from build123d import *

# Parameters (mm, degrees)
SALIENTE_EXTRUIR1_DEPTH = 40
CROQUIS2_R              = 3
CORTAR_EXTRUIR1_DEPTH   = 10


with BuildPart() as part:
    # Croquis1 → Saliente-Extruir1 (new body)
    with BuildSketch(Plane(origin=(0, 0, 0), x_dir=(1, 0, 0), z_dir=(0, 1, 0))):
        with BuildLine():
            Line((6.013434035, -15.633333333), (31.013434035, -15.633333333))
            Line((31.013434035, -15.633333333), (31.013434035, -12.633333333))
            Line((31.013434035, -12.633333333), (15.504802123, -12.633333333))
            ThreePointArc((15.504802123, -12.633333333), (0, 20), (-15.504802123, -12.633333333))
            Line((-15.504802123, -12.633333333), (-31.013434035, -12.633333333))
            Line((-31.013434035, -12.633333333), (-31.013434035, -15.633333333))
            Line((-31.013434035, -15.633333333), (-6.013434035, -15.633333333))
            ThreePointArc((-6.013434035, -15.633333333), (0, 16.75), (6.013434035, -15.633333333))
        make_face()
    extrude(amount=SALIENTE_EXTRUIR1_DEPTH)

    # Croquis2 → Cortar-Extruir1 (cut)
    with BuildSketch(Plane(origin=(0, 0, 12.633333333), x_dir=(-1, 0, 0), z_dir=(0, 0, -1))):
        with Locations((25.013434035, 8.154431535)):
            Circle(CROQUIS2_R)
        with Locations((25.013434035, 20.154431535)):
            Circle(CROQUIS2_R)
        with Locations((25.013434035, 32.154431535)):
            Circle(CROQUIS2_R)
        with Locations((-25.013434035, 32.154431535)):
            Circle(CROQUIS2_R)
        with Locations((-25.013434035, 8.154431535)):
            Circle(CROQUIS2_R)
        with Locations((-25.013434035, 20.154431535)):
            Circle(CROQUIS2_R)
    extrude(amount=-CORTAR_EXTRUIR1_DEPTH, mode=Mode.SUBTRACT)


solid = part.part
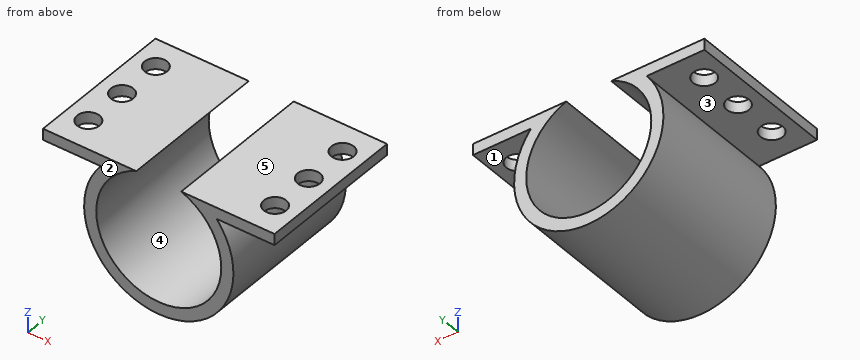
Could you check a few things on this model? Use its own coordinates, in mm. Face numbers are marked on the shaded views. A direction names the side the tool comes from. Coordinates: 2 decimals unless noted, no trailing zeros. Loops run counter-clockwise (first coordinate to the right, second up) from the corner with the lowest first, then second, coordinate; pieces in that order, holes last.
1. I need wall thicknesses on L1, parallel to X at y = 28, z = 0.5; L2, parallel to Z at x = -24.5, y = 4; L3, parallel to Z at x = 14.5, y = 15.5. Which ranges of each line are inside material? Lowest first, please.
2. For P1, Ø1.5, axis at y = 21, z = -8, coming from the +X side; P2, Ø17, axis at x = -21, y = 25.5, coming from the -Z side; P3, Ø7, axis at x = 25.01, y = 20.15, coming from the +Z side; P4, Ø5, axis at y = 25.5, z = -9, coming from the -X side, each with a flat end and sliding along its axis, tell me the tip position at first contact or that it passes through.
3. Imagine slicing it at D-D (y = 27). Please give me the cut outline in (x, z), and give its area (3 significant figures).
4. We'd pull the mould along X, two halves only. Please class the marked faces 4 and 5: released by +X, released by -X, zero draft, split by the parting line, or undercut.
5. Imagine slicing it at C-C (y = 9). Please give me the cut outline in (x, z).
6. For the marked faces 1, 2 and 3, which set-ups out of +Z, -Z, +X, -X, +Y, -Y let a thin tool reach every point of the face, with its end or its side?
7. Imagine slicing it at B-B (x = -14). Please give me the cut outline in (y, z), and give its area (3 significant figures).
8. Imagine slicing it at A-A (z = 0). Please give me the cut outline in (x, y).
Computed values:
1. L1: x = -19.99 to -16.74, 16.74 to 19.99
1. L2: z = 12.63 to 15.63
1. L3: z = -13.77 to -8.39, 8.39 to 15.63
2. P1: stops at x = 18.64
2. P2: stops at z = -15.61
2. P3: stops at z = 15.63
2. P4: stops at x = -18.91
3. outline: (-31.01, 12.63) - (-15.5, 12.63) arc R20 ccw (long way) to (15.5, 12.63) - (31.01, 12.63) - (31.01, 15.63) - (6.01, 15.63) arc R16.75 cw (long way) to (-6.01, 15.63) - (-31.01, 15.63) - close
3. area: 411 mm2
4. face 4: undercut
4. face 5: zero draft
5. outline: (-31.01, 12.63) - (-27.89, 12.63) - (-27.89, 15.63) - (-31.01, 15.63) - close; (-22.14, 12.63) - (-15.5, 12.63) arc R20 ccw (long way) to (15.5, 12.63) - (22.14, 12.63) - (22.14, 15.63) - (6.01, 15.63) arc R16.75 cw (long way) to (-6.01, 15.63) - (-22.14, 15.63) - close; (27.89, 12.63) - (31.01, 12.63) - (31.01, 15.63) - (27.89, 15.63) - close
6. face 1: +X, +Y, -Y
6. face 2: +Z, -Z, +X, -X, -Y
6. face 3: -X, +Y, -Y
7. outline: (0, -14.28) - (40, -14.28) - (40, -9.2) - (0, -9.2) - close; (0, 9.2) - (40, 9.2) - (40, 15.63) - (0, 15.63) - close
7. area: 461 mm2
8. outline: (-20, 0) - (-16.75, 0) - (-16.75, 40) - (-20, 40) - close; (16.75, 0) - (20, 0) - (20, 40) - (16.75, 40) - close
